Here's the drawing with two shaded views (mm, measured from the low corner). I have some questions. Coordinates: 2 decimals unless noted, no trailing zeros. Order: outer loops, then holes, each group sorted by start corner. A loop starts at its lowest first (then second) coordinate and runs counter-clockwise, first axis right, second up. Notation, with made-up numbers: M -21,-20 L -2,-20 A37 ccw -2,16 Z; hole C 63,16 d2. An arc over 180 degrees is marked long. Put each result on its own line as item: value. Start each with the question number.
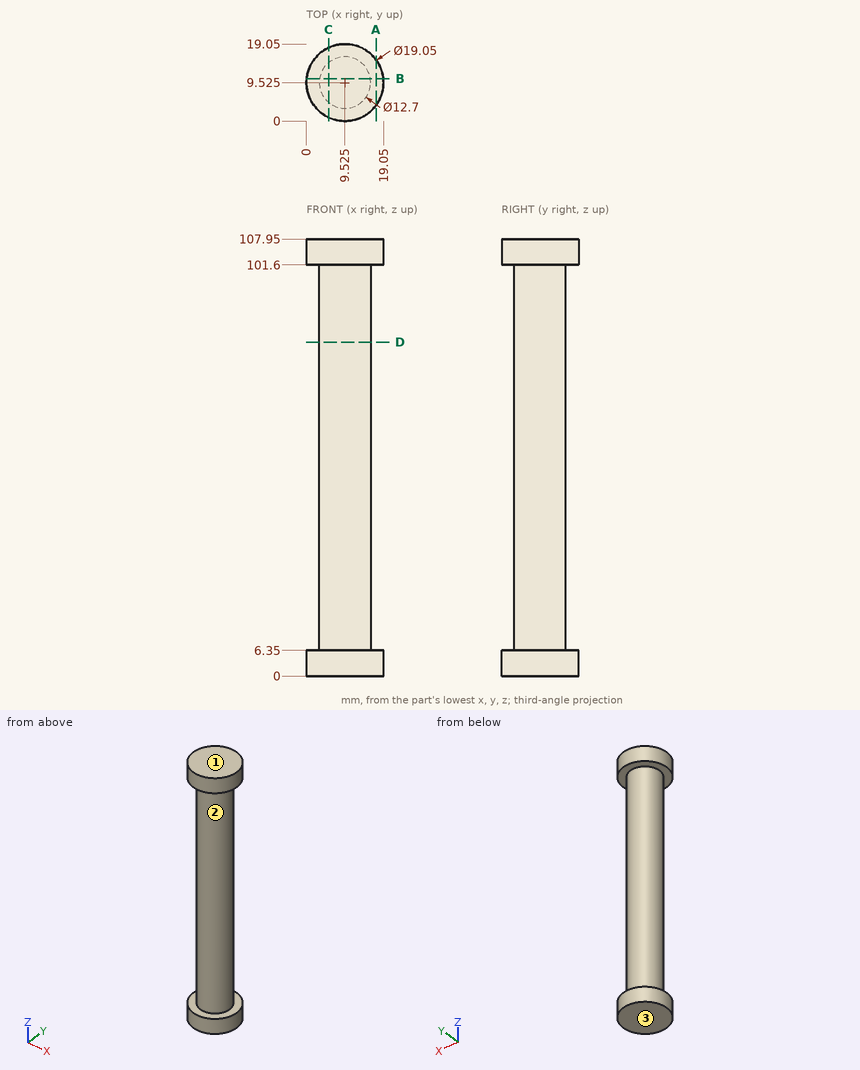
Item 1: If we mould it in two halves opening along Z, with no side actions, what happens to the marked faces 1, 2 and 3? For each: released by +Z, released by -Z, zero draft, split by the parting line, or undercut.
Item 2: I need wall thicknesses on probe 1 along Z at (x, y) = (8.5, 17); probe 2 along Y at (x, z) = (9, 69); probe 3 along X at (y, z) = (4.25, 98). Which ranges of each line are inside material? Lowest first, please.
Item 3: For pin 1 Ø6 at (y, z) = (9.5, 65.5) entering from -X (3 decimals); pin 2 Ø1.5 at (x, z) = (7, 76.5) entering from -Y; pin 3 Ø10 at (x, z) = (7, 78) entering from +Y (3 decimals), each with a flat end and sliding along its axis, tell me the tip position at first contact or that it passes through.
Item 4: If we section it at B-B on y = 10.5: Write out the boundary of the cut face in (x, z).
Item 5: If we section it at C-C on x = 5.5: Write out the boundary of the cut face in (y, z).
Item 6: If we section it at D-D on z = 82.5: Write out the boundary of the cut face in (x, y) (3 decimals), then the cut area to 3 significant figures.
Item 7: If we section it at A-A on x = 17.25: Write out the boundary of the cut face in (y, z).
Geometry check:
1. face 1: released by +Z
1. face 2: undercut
1. face 3: released by -Z
2. probe 1: z = 0 to 6.35, 101.6 to 107.95
2. probe 2: y = 3.2 to 15.85
2. probe 3: x = 5.99 to 13.06
3. pin 1: stops at x = 3.175
3. pin 2: stops at y = 3.43
3. pin 3: stops at y = 15.875
4. outline: M 0.05,0 L 19,0 L 19,6.35 L 15.8,6.35 L 15.8,101.6 L 19,101.6 L 19,107.95 L 0.05,107.95 L 0.05,101.6 L 3.25,101.6 L 3.25,6.35 L 0.05,6.35 Z
5. outline: M 0.89,0 L 18.16,0 L 18.16,6.35 L 14.44,6.35 L 14.44,101.6 L 18.16,101.6 L 18.16,107.95 L 0.89,107.95 L 0.89,101.6 L 4.61,101.6 L 4.61,6.35 L 0.89,6.35 Z
6. outline: C 9.525,9.525 d12.7
6. area: 127 mm²
7. outline: M 3.95,0 L 15.1,0 L 15.1,6.35 L 3.95,6.35 Z; M 3.95,101.6 L 15.1,101.6 L 15.1,107.95 L 3.95,107.95 Z
